from build123d import *

# Parameters (mm, degrees)
F0_W     = 50
F0_H     = 10
F0_H_2   = 15
F1_DEPTH = 1000


with BuildPart() as f1:
    # F0 (on Front) → F1 (new body)
    with BuildSketch(Plane.XZ):
        with Locations((-60, 38.86711)):
            Rectangle(F0_W, F0_H)
        Polygon((-25, 43.86711), (-35, 43.86711), (-35, 33.86711), (-35, -7.5), (-25, -7.5), (-25, 7.5), align=None)
        Rectangle(F0_W, F0_H_2)
        Polygon((25, 43.86711), (25, 7.5), (25, -7.5), (35, -7.5), (35, 33.86711), (35, 43.86711), align=None)
        with Locations((60, 38.86711)):
            Rectangle(F0_W, F0_H)
    extrude(amount=F1_DEPTH)


solid = f1.part
Part model, mm, in its own coordinate system. A direction names the side the tool comes from. Give positions to 0.01 mm unless a question says otherwise; leave off trailing zeros. Write each loop counter-clockwise with the first axis right and the second up, starting at its lowest first coordinate (ties: lowest second). Pieces come first, ordered by that corner, then holes.
1) Cut at B-B on y = -532. Write the cut outline in (x, z).
Resolved:
outline: (-85, 33.87) - (-35, 33.87) - (-35, -7.5) - (35, -7.5) - (35, 33.87) - (85, 33.87) - (85, 43.87) - (25, 43.87) - (25, 7.5) - (-25, 7.5) - (-25, 43.87) - (-85, 43.87) - close
2) Cut at C-C on x = -59.5. Write the cut outline in (y, z), then the cut area to 3 significant figures.
Resolved:
outline: (-1000, 33.87) - (0, 33.87) - (0, 43.87) - (-1000, 43.87) - close
area: 10,000 mm2
3) Pin check, flat tips, straight feed: pin 1 (3 mm diameter, centred on y = -788.5, z = 26.5, fed in from -X); pin 2 (4 mm diameter, centred on x = 58, y = -415.5, fed in from -Z); pin 3 (11 mm diameter, centred on y = -673, z = 21.5, fed in from +X). Stop position of each tip, or through.
Resolved:
pin 1: stops at x = -35
pin 2: stops at z = 33.87
pin 3: stops at x = 35
4) Cut at A-A on z = 18.5. Write the cut outline in (x, y).
Resolved:
outline: (-35, -1000) - (-25, -1000) - (-25, 0) - (-35, 0) - close; (25, -1000) - (35, -1000) - (35, 0) - (25, 0) - close
5) Probe L1, parallel to X at y = -486, z = 12; L2, parallel to X at y = -548.5, z = 36; L3, parallel to Z at x = -47.5, y = -480. List the from-to ranges inside material, lowest first.
Resolved:
L1: x = -35 to -25, 25 to 35
L2: x = -85 to -25, 25 to 85
L3: z = 33.87 to 43.87
6) Two-plate mould, pull along X, no slides. Class faces 6 (the face through (0, -493, -7.5)), 7 (the face through (-25, -493, 25)), 8 (the face through (35, -493, 13)): released by +X, released by -X, zero draft, split by the parting line, or undercut.
Resolved:
face 6: zero draft
face 7: undercut
face 8: released by +X
7) Which spindle directions (+Z, -Z, +X, -X, +Y, -Y) get a long thin tool onto all of the face, cutting with end or side? Do faces 1 (the face through (-55, -493, 43.867)), 2 (the face through (0, 0, 7)), 3 (the face through (60, -493, 33.867)), 4 (the face through (0, -493, 7.5)), 5 (the face through (-60, -493, 33.867)). Say none if no direction does.
Resolved:
face 1: +Z, +X, -X, +Y, -Y
face 2: +Z, -Z, +X, -X, +Y
face 3: -Z, +X, +Y, -Y
face 4: +Z, +Y, -Y
face 5: -Z, -X, +Y, -Y
